The model under review builds one solid part; all positions refer to its coordinate system, in mm. Give positions to 0.01 mm unless a question says otherwise; leave off trailing zeros. Order: outer loops, then holes, each group sorted by start corner. A loop starts at its lowest first (then second) coordinate and runs counter-clockwise, first axis right, second up. Notation, with made-up numbers: (70.25, 17.5) - (90.25, 17.5) arc R17 cw to (90.25, 43.5) - close; hole circle Ø8 at (-23.75, -9). An arc over 180 degrees is marked (long way). Put each result on its own line as item: value.
```python
from build123d import *

# Parameters (mm, degrees)
SKETCH_1_W      = 29
SKETCH_1_H      = 18
SKETCH_1_R      = 1.7
EXTRUDE_1_DEPTH = 2


with BuildPart() as part:
    # 草图1 → 凸台-拉伸1 (new body)
    with BuildSketch(Plane.XY):
        with Locations((14.5, 9)):
            Rectangle(SKETCH_1_W, SKETCH_1_H)
        with Locations((21.5, 7)):
            Circle(SKETCH_1_R, mode=Mode.SUBTRACT)
        with Locations(Location((7.5, 7, 0), (0, 0, 180))):
            Circle(SKETCH_1_R, mode=Mode.SUBTRACT)
    extrude(amount=EXTRUDE_1_DEPTH)


solid = part.part
```
(1) The part is to be moulded in two halves that separate along Y. For faces 1 (the cylindrical face through (22.3, 5.5, 1)), 2 (the flat face through (14, 0, 1)), 3 (the cylindrical face through (7.87, 8.66, 0.99)), 4 (the flat face through (14, 9, 0)), say which applies: pulls with the +Y half, pulls with the -Y half, needs draft (parallel to the pull), parting line crosses it, or undercut.
The answers:
face 1: undercut
face 2: pulls with the -Y half
face 3: undercut
face 4: needs draft
(2) Take a section at B-B, the plane x = 21.5. Write out the cut boundary in (y, z), then the cut area to 3 significant figures.
The answers:
outline: (0, 0) - (5.3, 0) - (5.3, 2) - (0, 2) - close; (8.7, 0) - (18, 0) - (18, 2) - (8.7, 2) - close
area: 29.2 mm^2
(3) Clearance check with a flat-ended pin moving along its axis: pin 1 Ø3 at (x, y) = (21.5, 7) entering from +Z. State where the tip first meets the part, or that it passes through.
The answers:
pin 1: through
(4) Wall thickness on L1, parallel to Y at x = 21.5, z = 0.5; L2, parallel to Y at x = 23, z = 1.9: over which ranges is each line inside the solid? List them lowest first.
The answers:
L1: 0 to 5.3, 8.7 to 18
L2: 0 to 6.2, 7.8 to 18
(5) Take a section at C-C, the plane z = 0.9. Write out the cut boundary in (x, y), then the cut area to 3 significant figures.
The answers:
outline: (0, 0) - (29, 0) - (29, 18) - (0, 18) - close; hole circle Ø3.4 at (7.5, 7); hole circle Ø3.4 at (21.5, 7)
area: 504 mm^2
(6) Take a section at A-A, the plane y = 7. Write out the cut boundary in (x, z).
The answers:
outline: (0, 0) - (5.8, 0) - (5.8, 2) - (0, 2) - close; (9.2, 0) - (19.8, 0) - (19.8, 2) - (9.2, 2) - close; (23.2, 0) - (29, 0) - (29, 2) - (23.2, 2) - close
